The model under review builds one solid part; all positions refer to its coordinate system, in mm. A direction names the side the tool comes from. Round coordinates to 2 decimals unless told otherwise and drop trailing zeros. Loops run counter-clockwise (first coordinate to the right, second up) from the corner with the lowest first, then second, coordinate; pieces in that order, holes last. Notation, with made-up numbers: M -0.75,-26 L 42.25,-26 A21 ccw 42.25,-5 Z; hole C 0,20.25 d3. An arc over 180 degrees is marked long. Answer as a JSON object with one key per item and string values. Group by question number.
Item 1: Tool access review of faces 4 (the face through (7, 8, 2)), 5 (the face through (-22.75, -15.68, 0.81)), 6 (the face through (33, 1, 30)), 7 (the face through (-33, -1, 30)): name each direction out of +Z, -Z, +X, -X, +Y, -Y from which nothing blocks a thin tool from reaching the whole face with its end or side.
Item 2: To check wall thickness, follow line 1 (Y direction, x = 0, z = 1.05); line 2 (X direction, y = 1, z = -8); line 3 (Y direction, x = 13.01, z = 0.8). State the ranges of each line that lie inside material, in increasing order.
Item 3: Consider section A-A (x = 21.85). Give the boundary of the cut face in (y, z), and give its area (3 significant figures).
Item 4: Consider section D-D (z = 28.5). State how many separate pieces and enclosed holes the cut face has, and give its area (3 significant figures).
Item 5: Insertion check: P1, Ø12, axis at x = 21, z = 25.5, coming from the +Y side; P2, Ø8, axis at y = 0, z = 28.5, coming from the +X side; P3, Ø2, axis at x = -8.5, y = -7.5, coming from the +Z side; P4, Ø2.5, axis at x = 21.85, y = 0, coming from the +Z side. Each pin has a flat end and moves straight along its axis. Give the tip position at first contact, or say it passes through.
Item 6: The part is to be moulded in two halves that separate along Y. For faces 1 (the face through (-30, 12, 35.5)), 2 (the face through (1, -33, 30)), 3 (the face through (22.666, 15.595, 1.188)), say which applies: +Y half, -Y half, draft (parallel to the pull), parting line (faces both ways), or undercut.
Item 7: Consider section C-C (z = 18.5). Give the boundary of the cut face in (x, y).
```python
from build123d import *
from build123d.topology import SkipClean

# Parameters (mm, degrees)
SKETCH1_R               = 33.51
BOSS_EXTRUDE1_DEPTH     = 2
SKETCH2_R               = 33.51
SKETCH2_R_2             = 32
BOSS_EXTRUDE2_DEPTH     = 23.5
SKETCH3_R               = 1.5
CUT_EXTRUDE1_DEPTH      = 54.815334246
SKETCH4_R               = 10
CUT_EXTRUDE2_DEPTH      = 53.896977229
CUT_EXTRUDE3_DEPTH      = 53.896977229
CUT_EXTRUDE3_DEPTH_BACK = 10
BOSS_EXTRUDE3_START     = 10
SKETCH6_R               = 33.51
SKETCH6_R_2             = 32
BOSS_EXTRUDE3_DEPTH     = 10
FILLET1_R               = 1
SKETCH7_R               = 33.51
SKETCH7_R_2             = 32
BOSS_EXTRUDE4_DEPTH     = 10
CUT_EXTRUDE4_DEPTH      = 10
SKETCH9_R               = 1.5
CUT_EXTRUDE5_DEPTH      = 10
CIRPATTERN1_COUNT       = 4
SKETCH11_R              = 2.5
CUT_EXTRUDE6_DEPTH      = 1
CIRPATTERN2_COUNT       = 4


with BuildPart() as part:
    # Sketch1 → Boss-Extrude1 (new body)
    with BuildSketch(Plane.XY):
        Circle(SKETCH1_R)
    extrude(amount=BOSS_EXTRUDE1_DEPTH)

    # Sketch2 → Boss-Extrude2 (add)
    with BuildSketch(Plane.XY.offset(2)):
        Circle(SKETCH2_R)
        Circle(SKETCH2_R_2, mode=Mode.SUBTRACT)
    extrude(amount=BOSS_EXTRUDE2_DEPTH)

    # Sketch3 → Cut-Extrude1 (cut, through all)
    with BuildSketch(Plane(origin=(0, 0, 0), x_dir=(-1, 0, 0), z_dir=(0, 0, -1))):
        with Locations((21.85, 0)):
            Circle(SKETCH3_R)
        with Locations((13.01, 0)):
            Circle(SKETCH3_R)
        with Locations((0, -21.85)):
            Circle(SKETCH3_R)
        with Locations((0, -13.01)):
            Circle(SKETCH3_R)
        with Locations((-21.85, 0)):
            Circle(SKETCH3_R)
        with Locations((-13.01, 0)):
            Circle(SKETCH3_R)
        with Locations((0, 21.85)):
            Circle(SKETCH3_R)
        with Locations((0, 13.01)):
            Circle(SKETCH3_R)
    extrude(amount=-CUT_EXTRUDE1_DEPTH, mode=Mode.SUBTRACT)

    # Sketch4 → Cut-Extrude2 (cut, through all)
    with BuildSketch(Plane.XY.offset(2)):
        Circle(SKETCH4_R)
    extrude(amount=-CUT_EXTRUDE2_DEPTH, mode=Mode.SUBTRACT)

    # Sketch5 → Cut-Extrude3 (cut, two sides: drawn at the far end of the back side and taken through both)
    with BuildSketch(Plane.XY.offset(2).offset(-CUT_EXTRUDE3_DEPTH_BACK)):
        with BuildLine():
            Line((-12.464466094, 19.535533906), (-18.813962733, 25.885030545))
            ThreePointArc((-18.813962733, 25.885030545), (-22.627416998, 22.627416998), (-25.885030545, 18.813962733))
            Line((-25.885030545, 18.813962733), (-19.535533906, 12.464466094))
            Line((-19.535533906, 12.464466094), (-12.464466094, 19.535533906))
        make_face()
        with BuildLine():
            Line((19.535533906, 12.464466094), (25.885030545, 18.813962733))
            ThreePointArc((25.885030545, 18.813962733), (22.627416998, 22.627416998), (18.813962733, 25.885030545))
            Line((18.813962733, 25.885030545), (12.464466094, 19.535533906))
            Line((12.464466094, 19.535533906), (19.535533906, 12.464466094))
        make_face()
        with BuildLine():
            Line((-19.535533906, -12.464466094), (-25.885030545, -18.813962733))
            ThreePointArc((-25.885030545, -18.813962733), (-22.627416998, -22.627416998), (-18.813962733, -25.885030545))
            Line((-18.813962733, -25.885030545), (-12.464466094, -19.535533906))
            Line((-12.464466094, -19.535533906), (-19.535533906, -12.464466094))
        make_face()
        with BuildLine():
            ThreePointArc((18.813962733, -25.885030545), (22.627416998, -22.627416998), (25.885030545, -18.813962733))
            Line((25.885030545, -18.813962733), (19.535533906, -12.464466094))
            Line((19.535533906, -12.464466094), (12.464466094, -19.535533906))
            Line((12.464466094, -19.535533906), (18.813962733, -25.885030545))
        make_face()
    extrude(amount=CUT_EXTRUDE3_DEPTH + CUT_EXTRUDE3_DEPTH_BACK, mode=Mode.SUBTRACT)

    # Sketch6 → Boss-Extrude3 (add)
    with BuildSketch(Plane(origin=(0, 0, 0), x_dir=(-1, 0, 0), z_dir=(0, 0, -1)).offset(BOSS_EXTRUDE3_START)):
        Circle(SKETCH6_R)
        Circle(SKETCH6_R_2, mode=Mode.SUBTRACT)
    extrude(amount=-BOSS_EXTRUDE3_DEPTH)

    # Fillet1
    # the kernel refuses this fillet: 1 mm, written as the material it adds along each edge
    with BuildSketch(Plane(origin=(0, 0, 0), x_dir=(-1, 0, 0), z_dir=(0, -1, 0))) as fillet1_piece_1_section:
        with BuildLine():
            CenterArc((32 - FILLET1_R, FILLET1_R), FILLET1_R, 270, 90)
            Line((32 - FILLET1_R, 0), (32, 0))
            Line((32, 0), (32, FILLET1_R))
        make_face()
    fillet1_piece_1 = revolve(axis=Axis((0, 0, 0), (0, 0, -1)), revolution_arc=40.487221235, mode=Mode.PRIVATE)
    fillet1_piece_1 = split(fillet1_piece_1, bisect_by=Plane(origin=(-23.520787378, 16.449719566, -0.28073515), z_dir=(-0.707106781186554, -0.707106781186541, 0)), keep=Keep.TOP, mode=Mode.PRIVATE)
    add(fillet1_piece_1)
    with BuildSketch(Plane(origin=(0, 0, 0), x_dir=(0.6492899007478581, -0.7605410079587009, 0), z_dir=(0.7605410079587009, 0.6492899007478581, 0))) as fillet1_piece_2_section:
        with BuildLine():
            CenterArc((32 - FILLET1_R, FILLET1_R), FILLET1_R, 270, 90)
            Line((32 - FILLET1_R, 0), (32, 0))
            Line((32, 0), (32, FILLET1_R))
        make_face()
    fillet1_piece_2 = revolve(axis=Axis((0, 0, 0), (0, 0, -1)), revolution_arc=80.976169612, mode=Mode.PRIVATE)
    fillet1_piece_2 = split(fillet1_piece_2, bisect_by=Plane(origin=(12.325678578, -19.39674639, -0.277575032), z_dir=(-0.7071067811865488, -0.7071067811865462, 0)), keep=Keep.TOP, mode=Mode.PRIVATE)
    fillet1_piece_2 = split(fillet1_piece_2, bisect_by=Plane(origin=(-12.325678578, -19.39674639, -0.277575032), z_dir=(0.7071067811865432, -0.7071067811865519, 0)), keep=Keep.TOP, mode=Mode.PRIVATE)
    add(fillet1_piece_2)
    with BuildSketch(Plane(origin=(0, 0, 0), x_dir=(0.7605410079586984, 0.6492899007478611, 0), z_dir=(-0.6492899007478611, 0.7605410079586984, 0))) as fillet1_piece_3_section:
        with BuildLine():
            CenterArc((32 - FILLET1_R, FILLET1_R), FILLET1_R, 270, 90)
            Line((32 - FILLET1_R, 0), (32, 0))
            Line((32, 0), (32, FILLET1_R))
        make_face()
    fillet1_piece_3 = revolve(axis=Axis((0, 0, 0), (0, 0, -1)), revolution_arc=80.976169612, mode=Mode.PRIVATE)
    fillet1_piece_3 = split(fillet1_piece_3, bisect_by=Plane(origin=(19.39674639, -12.325678578, -0.277575032), z_dir=(0.7071067811865495, 0.7071067811865457, 0)), keep=Keep.TOP, mode=Mode.PRIVATE)
    fillet1_piece_3 = split(fillet1_piece_3, bisect_by=Plane(origin=(19.39674639, 12.325678578, -0.277575032), z_dir=(0.7071067811865487, -0.7071067811865466, 0)), keep=Keep.TOP, mode=Mode.PRIVATE)
    add(fillet1_piece_3)
    with BuildSketch(Plane(origin=(0, 0, 0), x_dir=(-0.6492899007478526, 0.7605410079587055, 0), z_dir=(-0.7605410079587055, -0.6492899007478526, 0))) as fillet1_piece_4_section:
        with BuildLine():
            CenterArc((32 - FILLET1_R, FILLET1_R), FILLET1_R, 270, 90)
            Line((32 - FILLET1_R, 0), (32, 0))
            Line((32, 0), (32, FILLET1_R))
        make_face()
    fillet1_piece_4 = revolve(axis=Axis((0, 0, 0), (0, 0, -1)), revolution_arc=80.976169612, mode=Mode.PRIVATE)
    fillet1_piece_4 = split(fillet1_piece_4, bisect_by=Plane(origin=(-12.325678578, 19.39674639, -0.277575032), z_dir=(0.7071067811865538, 0.7071067811865415, 0)), keep=Keep.TOP, mode=Mode.PRIVATE)
    fillet1_piece_4 = split(fillet1_piece_4, bisect_by=Plane(origin=(12.325678578, 19.39674639, -0.277575032), z_dir=(-0.707106781186548, 0.707106781186547, 0)), keep=Keep.TOP, mode=Mode.PRIVATE)
    add(fillet1_piece_4)
    with BuildSketch(Plane(origin=(0, 0, 0), x_dir=(-0.7605507940779602, -0.6492784376732254, 0), z_dir=(0.6492784376732254, -0.7605507940779602, 0))) as fillet1_piece_5_section:
        with BuildLine():
            CenterArc((32 - FILLET1_R, FILLET1_R), FILLET1_R, 270, 90)
            Line((32 - FILLET1_R, 0), (32, 0))
            Line((32, 0), (32, FILLET1_R))
        make_face()
    fillet1_piece_5 = revolve(axis=Axis((0, 0, 0), (0, 0, -1)), revolution_arc=40.487221235, mode=Mode.PRIVATE)
    fillet1_piece_5 = split(fillet1_piece_5, bisect_by=Plane(origin=(-23.520787379, -16.449719567, -0.280735148), z_dir=(-0.7071067811865441, 0.707106781186551, 0)), keep=Keep.TOP, mode=Mode.PRIVATE)
    add(fillet1_piece_5)

    # Sketch7 → Boss-Extrude4 (add)
    with SkipClean():  # the faces are left unmerged after this step: merging them gives an invalid solid
        with BuildSketch(Plane.XY.offset(25.5)):
            with Locations(Location((0, 0, 0), (0, 0, 180))):
                Circle(SKETCH7_R)
            with Locations(Location((0, 0, 0), (0, 0, 180))):
                Circle(SKETCH7_R_2, mode=Mode.SUBTRACT)
        extrude(amount=BOSS_EXTRUDE4_DEPTH)
    add(part.part.scale(1), mode=Mode.REPLACE)  # the faces are merged on a copy

    # Sketch8 → Cut-Extrude4 (cut)
    with BuildSketch(Plane.XY.offset(35.5)):
        Polygon((32, 0), (32, 5), (31.606961259, 5), (31.606961259, -5), (32, -5), align=None)
        Polygon((-5, -32), (0, -32), (5, -32), (5, -31.606961259), (-5, -31.606961259), align=None)
        Polygon((-32, 5), (-32, 0), (-32, -5), (-31.606961259, -5), (-31.606961259, 5), align=None)
        Polygon((5, 32), (0, 32), (-5, 32), (-5, 31.606961259), (5, 31.606961259), align=None)
    extrude(amount=-CUT_EXTRUDE4_DEPTH, mode=Mode.SUBTRACT)

    # Sketch9 → Cut-Extrude5 (cut)
    with BuildSketch(Plane.XZ.offset(-32)):
        with Locations((0, 28.5)):
            Circle(SKETCH9_R)
    cut_extrude5 = extrude(amount=-CUT_EXTRUDE5_DEPTH, mode=Mode.SUBTRACT)

    # CirPattern1: Cut-Extrude5 ×4 about axis
    cirpattern1_axis = Axis((0, 0, 25.5), (0, 0, -1))
    for i in range(1, CIRPATTERN1_COUNT):
        add(cut_extrude5.rotate(cirpattern1_axis, i * 360 / CIRPATTERN1_COUNT), mode=Mode.SUBTRACT)

    # Sketch11 → Cut-Extrude6 (cut)
    with BuildSketch(Plane(origin=(0, 34, 0), x_dir=(-1, 0, 0), z_dir=(0, -1, 0))):
        with Locations((0, -28.5)):
            Circle(SKETCH11_R)
    cut_extrude6 = extrude(amount=CUT_EXTRUDE6_DEPTH, mode=Mode.SUBTRACT)

    # CirPattern2: Cut-Extrude6 ×4 about axis
    cirpattern2_axis = Axis((0, 0, 0), (0, 0, 1))
    for i in range(1, CIRPATTERN2_COUNT):
        add(cut_extrude6.rotate(cirpattern2_axis, i * 360 / CIRPATTERN2_COUNT), mode=Mode.SUBTRACT)


solid = part.part
```
Geometry results:
{
 "1": {"face 4": "+Z", "face 5": "+Z, -Z", "face 6": "+X", "face 7": "-X"},
 "2": {"line 1": "y = -33.51 to -23.35, -20.35 to -14.51, -11.51 to -10, 10 to 11.51, 14.51 to 20.35, 23.35 to 33.51", "line 2": "x = -33.5 to -31.98, 31.98 to 33.5", "line 3": "y = -30.88 to -20.08, -18.99 to -1.5, 1.5 to 18.99, 20.08 to 30.88"},
 "3": {"outline": "M -25.41,-10 L -23.38,-10 L -23.38,35.5 L -25.41,35.5 Z; M -14.78,0 L -1.5,0 L -1.5,2 L -14.78,2 Z; M 1.5,0 L 14.78,0 L 14.78,2 L 1.5,2 Z; M 23.38,-10 L 25.41,-10 L 25.41,35.5 L 23.38,35.5 Z", "area": "238 mm^2"},
 "4": {"separate pieces": "4", "enclosed holes": "0", "area": "284 mm^2"},
 "5": {"P1": "stops at y = 29.97", "P2": "stops at x = 33.51", "P3": "stops at z = 2", "P4": "passes through"},
 "6": {"face 1": "draft", "face 2": "-Y half", "face 3": "undercut"},
 "7": {"outline": "C 0,0 d67.02; hole C 0,0 d64"}
}
